```python
from build123d import *

# Parameters (mm, degrees)
BOSS_EXTRUDE1_DEPTH = 10
SKETCH4_W           = 55
SKETCH4_H           = 46
CUT_EXTRUDE1_DEPTH  = 11
SKETCH5_R           = 3
SKETCH5_W           = 50
SKETCH5_H           = 50
CUT_EXTRUDE2_DEPTH  = 11
SKETCH6_R           = 4
CUT_EXTRUDE4_DEPTH  = 5
SKETCH7_R           = 2.5
CUT_EXTRUDE5_DEPTH  = 6
FILLET1_R           = 3
SKETCH8_R           = 4
CUT_EXTRUDE6_DEPTH  = 5


with BuildPart() as part:
    # Sketch3 → Boss-Extrude1 (new body)
    with BuildSketch(Plane(origin=(0, 0, 0), x_dir=(1, 0, 0), z_dir=(0, 1, 0))):
        Polygon((0, 0), (0, 70), (120, 70), (125, 65), (125, 5), (119.666666667, 0), align=None)
    extrude(amount=BOSS_EXTRUDE1_DEPTH)

    # Sketch4 → Cut-Extrude1 (cut, through all)
    with BuildSketch(Plane(origin=(0, 10, 0), x_dir=(1, 0, 0), z_dir=(0, 1, 0))):
        with Locations((27.5, 35)):
            Rectangle(SKETCH4_W, SKETCH4_H)
    extrude(amount=-CUT_EXTRUDE1_DEPTH, mode=Mode.SUBTRACT)

    # Sketch5 → Cut-Extrude2 (cut, through all)
    with BuildSketch(Plane(origin=(0, 10, 0), x_dir=(1, 0, 0), z_dir=(0, 1, 0))):
        with Locations((65, 60)):
            Circle(SKETCH5_R)
        with Locations((65, 10)):
            Circle(SKETCH5_R)
        with Locations((115, 10)):
            Circle(SKETCH5_R)
        with Locations((115, 60)):
            Circle(SKETCH5_R)
        with Locations((90, 35)):
            Rectangle(SKETCH5_W, SKETCH5_H)
        with BuildLine():
            Line((65, 57), (65, 60))
            Line((65, 60), (68, 60))
            ThreePointArc((68, 60), (62.878679656, 62.121320344), (65, 57))
        make_face()
        with BuildLine():
            Line((68, 60), (65, 60))
            Line((65, 60), (65, 57))
            ThreePointArc((65, 57), (67.121320344, 57.878679656), (68, 60))
        make_face()
        with BuildLine():
            ThreePointArc((118, 60), (115, 63), (112, 60))
            Line((112, 60), (115, 60))
            Line((115, 60), (115, 57))
            ThreePointArc((115, 57), (117.121320344, 57.878679656), (118, 60))
        make_face()
        with BuildLine():
            Line((115, 60), (112, 60))
            ThreePointArc((112, 60), (112.878679656, 57.878679656), (115, 57))
            Line((115, 57), (115, 60))
        make_face()
        with BuildLine():
            ThreePointArc((118, 10), (117.121320344, 12.121320344), (115, 13))
            Line((115, 13), (115, 10))
            Line((115, 10), (112, 10))
            ThreePointArc((112, 10), (115, 7), (118, 10))
        make_face()
        with BuildLine():
            Line((115, 10), (115, 13))
            ThreePointArc((115, 13), (112.878679656, 12.121320344), (112, 10))
            Line((112, 10), (115, 10))
        make_face()
        with BuildLine():
            ThreePointArc((68, 10), (67.121320344, 12.121320344), (65, 13))
            Line((65, 13), (65, 10))
            Line((65, 10), (68, 10))
        make_face()
        with BuildLine():
            Line((65, 10), (65, 13))
            ThreePointArc((65, 13), (62.878679656, 7.878679656), (68, 10))
            Line((68, 10), (65, 10))
        make_face()
    extrude(amount=-CUT_EXTRUDE2_DEPTH, mode=Mode.SUBTRACT)

    # Sketch6 → Cut-Extrude4 (cut)
    with BuildSketch(Plane(origin=(0, 10, 0), x_dir=(1, 0, 0), z_dir=(0, 1, 0))):
        with Locations((20, 64.59775654)):
            Circle(SKETCH6_R)
        with Locations((20, 5.658501093)):
            Circle(SKETCH6_R)
    extrude(amount=-CUT_EXTRUDE4_DEPTH, mode=Mode.SUBTRACT)

    # Sketch7 → Cut-Extrude5 (cut, through all)
    with BuildSketch(Plane(origin=(0, 5, 0), x_dir=(1, 0, 0), z_dir=(0, 1, 0))):
        with Locations((20, 64.59775654)):
            Circle(SKETCH7_R)
        with Locations((20, 5.658501093)):
            Circle(SKETCH7_R)
    extrude(amount=-CUT_EXTRUDE5_DEPTH, mode=Mode.SUBTRACT)

    # Fillet1
    fillet1_edges = [part.edges().sort_by_distance(p)[0] for p in [
        (55, 5, -58),
        (55, 5, -12),
    ]]
    fillet(fillet1_edges, radius=FILLET1_R)

    # Sketch8 → Cut-Extrude6 (cut)
    with BuildSketch(Plane(origin=(0, 10, 0), x_dir=(1, 0, 0), z_dir=(0, 1, 0))):
        with Locations((120, 50)):
            Circle(SKETCH8_R)
        with Locations((120, 20)):
            Circle(SKETCH8_R)
        with Locations((105, 65)):
            Circle(SKETCH8_R)
        with Locations((75, 65)):
            Circle(SKETCH8_R)
        with Locations((75, 5)):
            Circle(SKETCH8_R)
        with Locations((105, 5)):
            Circle(SKETCH8_R)
        with Locations((60, 50)):
            Circle(SKETCH8_R)
        with Locations((60, 20)):
            Circle(SKETCH8_R)
    extrude(amount=-CUT_EXTRUDE6_DEPTH, mode=Mode.SUBTRACT)


solid = part.part
```
Source: CAD feature listing. Evaluate the final solid. Frame: model axes, mm. A direction names the side the tool comes from. Coordinates: 2 decimals unless noted, no trailing zeros. Loops run counter-clockwise (first coordinate to the right, second up) from the corner with the lowest first, then second, coordinate; pieces in that order, holes last. Notation, with made-up numbers: (13.5, 4.5) -> (39.5, 4.5) arc R29 ccw to (39.5, 36.5) -> close; hole circle Ø6 at (24, 8.25). An arc over 180 degrees is marked (long way). One line per item, written item: value. Start each with the question number.
Q1. Contact query for a flat-ended pin moving along its axis: P1, Ø2.5, axis at x = 105.5, z = -64.5, coming from the +Y side. Output: stop coordinate, or through.
Q2. Section query D-D, the plane y = 7. Give the number of separate pieces and of enclosed holes in the cut face, and give its area (3 significant figures).
Q3. Line query: line 1 along X through (y, z) = (8.5, -50); line 2 along Z through (x, y) = (75, 7.4); line 3 along Z through (x, y) = (20, 2). Output: solid intervals per line, ascending.
Q4. Section query B-B, the plane z = -42.5. Return the cut outline in (x, y), and give its area (3 significant figures).
Q5. Mould query, pull axis Z, two halves, no side actions, for faces 1 (the face through (122.371, 4.93, -2.535)), 2 (the face through (63, 0, -35)), 3 (the face through (119.133, 7.535, -46.095)). Classes: pulls with the +Z half, pulls with the -Z half, needs draft (parallel to the pull), parting line crosses it, or undercut.
Q6. Section query A-A, the plane x = 40. Return the cut outline in (y, z).
Q7. Section query C-C, the plane x = 60. Return the cut outline in (y, z), and give its area (3 significant figures).
Q8. Set-up query: faces 4 (the face through (63.815, 7.535, -21.201)), 5 (the face through (0, 5, -6)), 6 (the face through (115, 5, -35)). Return all of +Z, -Z, +X, -X, +Y, -Y with unobstructed straight access to the full face (end or side cutting, diameter ignored); none if empty.
Results:
1. P1: y = 5
2. separate pieces: 1
2. enclosed holes: 11
2. area: 3,110 mm^2
3. line 1: 55 to 56, 64 to 65, 115 to 116, 124 to 125
3. line 2: -70 to -69, -61 to -60, -10 to -9, -1 to 0
3. line 3: -70 to -67.1, -62.1 to -58, -12 to -8.16, -3.16 to 0
4. outline: (55, 0) -> (65, 0) -> (65, 10) -> (55, 10) -> close; (115, 0) -> (125, 0) -> (125, 10) -> (115, 10) -> close
4. area: 200 mm^2
5. face 1: pulls with the +Z half
5. face 2: needs draft
5. face 3: undercut
6. outline: (0, -70) -> (10, -70) -> (10, -58) -> (0, -58) -> close; (0, -12) -> (10, -12) -> (10, 0) -> (0, 0) -> close
7. outline: (0, -70) -> (10, -70) -> (10, -54) -> (5, -54) -> (5, -46) -> (10, -46) -> (10, -24) -> (5, -24) -> (5, -16) -> (10, -16) -> (10, 0) -> (0, 0) -> close
7. area: 620 mm^2
8. face 4: +Y
8. face 5: +Z, -Z, -X, +Y, -Y
8. face 6: +Y, -Y
